Build history of the part. All positions in model axes, mm. A direction names the side the tool comes from. Coordinates: 2 decimals unless noted, no trailing zeros. Write each loop counter-clockwise with the first axis right and the second up, starting at its lowest first coordinate (ties: lowest second). Pieces come first, ordered by that corner, then holes.
```python
from build123d import *

# Parameters (mm, degrees)
BOSS_EXTRUDE1_DEPTH                                 = 15
FILLET1_R                                           = 6
CBORE_FOR_M6_HEX_SOCKET_HEAD_CAP_SCREW1_D           = 6.6
CBORE_FOR_M6_HEX_SOCKET_HEAD_CAP_SCREW1_CBORE_D     = 11
CBORE_FOR_M6_HEX_SOCKET_HEAD_CAP_SCREW1_CBORE_DEPTH = 6.4
SKETCH6_R                                           = 7
CUT_EXTRUDE3_DEPTH                                  = 16
SKETCH7_R                                           = 11
CUT_EXTRUDE4_DEPTH                                  = 11
TAP_DRILL_FOR_M5_TAP1_D                             = 4.2
TAP_DRILL_FOR_M5_TAP1_DEPTH                         = 10
TAP_DRILL_FOR_M5_TAP1_TIP                           = 1.2618073
FILLET4_R                                           = 14
FILLET5_R                                           = 10
CHAMFER1_SIZE                                       = 0.5


with BuildPart() as part:
    # Sketch1 → Boss-Extrude1 (new body)
    with BuildSketch(Plane.XY):
        with BuildLine():
            Line((-54.083500753, -8.556617627), (-54.083500753, -51.556617627))
            Line((-54.083500753, -51.556617627), (-21.808305332, -51.556617627))
            Line((-21.808305332, -51.556617627), (-10.687429148, -20.70518937))
            ThreePointArc((-10.687429148, -20.70518937), (19.416499247, 0.443382373), (49.520427642, -20.70518937))
            Line((49.520427642, -20.70518937), (60.641303826, -51.556617627))
            Line((60.641303826, -51.556617627), (92.916499247, -51.556617627))
            Line((92.916499247, -51.556617627), (92.916499247, 42.193382373))
            Line((92.916499247, 42.193382373), (-74.083500753, 42.193382373))
            Line((-74.083500753, 42.193382373), (-74.083500753, 144.193382373))
            Line((-74.083500753, 144.193382373), (-104.083500753, 144.193382373))
            Line((-104.083500753, 144.193382373), (-104.083500753, 41.443382373))
            Line((-104.083500753, 41.443382373), (-54.083500753, -8.556617627))
        make_face()
        with BuildLine():
            ThreePointArc((-93.483500753, 97.193382373), (-89.083500753, 101.593382373), (-84.683500753, 97.193382373))
            Line((-84.683500753, 97.193382373), (-84.683500753, 85.193382373))
            ThreePointArc((-84.683500753, 85.193382373), (-89.083500753, 80.793382373), (-93.483500753, 85.193382373))
            Line((-93.483500753, 85.193382373), (-93.483500753, 97.193382373))
        make_face(mode=Mode.SUBTRACT)
        with BuildLine():
            ThreePointArc((-93.483500753, 129.193382373), (-89.083500753, 133.593382373), (-84.683500753, 129.193382373))
            Line((-84.683500753, 129.193382373), (-84.683500753, 117.193382373))
            ThreePointArc((-84.683500753, 117.193382373), (-89.083500753, 112.793382373), (-93.483500753, 117.193382373))
            Line((-93.483500753, 117.193382373), (-93.483500753, 129.193382373))
        make_face(mode=Mode.SUBTRACT)
    extrude(amount=BOSS_EXTRUDE1_DEPTH)

    # Fillet1
    fillet1_edges = [part.edges().sort_by_distance(p)[0] for p in [
        (-21.808305332, -51.556617627, 7.5),
        (-54.083500753, -51.556617627, 7.5),
        (-104.083500753, 144.193382373, 7.5),
        (-74.083500753, 144.193382373, 7.5),
        (-74.083500753, 42.193382373, 7.5),
        (60.641303826, -51.556617627, 7.5),
    ]]
    fillet(fillet1_edges, radius=FILLET1_R)

    # CBORE for M6 Hex Socket Head Cap Screw1 (through all)
    with Locations(Plane.XY.offset(15)):
        with Locations((-31.583500753, -41.556617627), (-31.583500753, -21.556617627), (70.416499247, -41.556617627), (70.416499247, -21.556617627)):
            CounterBoreHole(CBORE_FOR_M6_HEX_SOCKET_HEAD_CAP_SCREW1_D / 2, CBORE_FOR_M6_HEX_SOCKET_HEAD_CAP_SCREW1_CBORE_D / 2, CBORE_FOR_M6_HEX_SOCKET_HEAD_CAP_SCREW1_CBORE_DEPTH)

    # Sketch6 → Cut-Extrude3 (cut, through all)
    with BuildSketch(Plane.XY.offset(15)):
        with Locations((78.916499247, 28.193382373)):
            Circle(SKETCH6_R)
    extrude(amount=-CUT_EXTRUDE3_DEPTH, mode=Mode.SUBTRACT)

    # Sketch7 → Cut-Extrude4 (cut)
    with BuildSketch(Plane.XY.offset(15)):
        with Locations((78.916499247, 28.193382373)):
            Circle(SKETCH7_R)
    extrude(amount=-CUT_EXTRUDE4_DEPTH, mode=Mode.SUBTRACT)

    # Tap Drill for M5 Tap1
    with Locations(Plane(origin=(0, 42.193382373, 0), x_dir=(1, 0, 0), z_dir=(0, 1, 0))):
        with Locations((-62.583500753, -7.5)):
            Hole(TAP_DRILL_FOR_M5_TAP1_D / 2, depth=TAP_DRILL_FOR_M5_TAP1_DEPTH)
            with Locations((0, 0, -(TAP_DRILL_FOR_M5_TAP1_DEPTH + TAP_DRILL_FOR_M5_TAP1_TIP / 2))):  # 118° drill point
                Cone(0, TAP_DRILL_FOR_M5_TAP1_D / 2, TAP_DRILL_FOR_M5_TAP1_TIP, mode=Mode.SUBTRACT)

    # Fillet4
    fillet4_edges = [part.edges().sort_by_distance(p)[0] for p in [
        (92.916499247, 42.193382373, 7.5),
    ]]
    fillet(fillet4_edges, radius=FILLET4_R)

    # Fillet5
    fillet5_edges = [part.edges().sort_by_distance(p)[0] for p in [
        (-54.083500753, -8.556617627, 7.5),
        (-104.083500753, 41.443382373, 7.5),
    ]]
    fillet(fillet5_edges, radius=FILLET5_R)

    # Chamfer1
    chamfer1_edges = [part.edges().sort_by_distance(p)[0] for p in [
        (64.916499247, -41.556617627, 15),
        (-37.083500753, -21.556617627, 15),
        (-37.083500753, -41.556617627, 15),
        (67.916499247, 28.193382373, 15),
        (-60.483500753, 42.193382373, 7.5),
        (88.815994184, 38.09287731, 15),
        (-79.083500753, 16.443382373, 15),
        (-104.083500753, 91.889450185, 15),
        (-103.322296078, 41.758683673, 15),
        (-54.844705428, -8.871918927, 15),
        (19.416499247, 0.443382373, 15),
        (54.366178458, -34.148224897, 15),
        (92.916499247, -11.681617627, 15),
        (-74.083500753, 93.193382373, 15),
        (5.416499247, 42.193382373, 15),
        (-89.083500753, 144.193382373, 15),
        (78.886457547, -51.556617627, 15),
        (-54.083500753, -29.127685439, 15),
        (-37.053459053, -51.556617627, 15),
        (-22.574349131, -50.466192801, 15),
        (61.407347625, -50.466192801, 15),
        (-52.32614144, -49.799258314, 15),
        (-102.32614144, 142.43602306, 15),
        (-75.840860066, 142.43602306, 15),
        (-72.32614144, 43.950741686, 15),
        (-15.533179964, -34.148224897, 15),
        (64.916499247, -21.556617627, 15),
    ]]
    chamfer(chamfer1_edges, length=CHAMFER1_SIZE)


solid = part.part
```
1. Flat gauge pins, fed straight in: pin 1 (3 mm diameter, centred on y = 19.5, z = 6, fed in from -X); pin 2 (11 mm diameter, centred on x = 75.5, y = 25.5, fed in from +Z); pin 3 (3.5 mm diameter, centred on x = 72, y = -21, fed in from +Z). Where does each tip first touch, or does it go through?
Computed values:
pin 1: stops at x = -83.64
pin 2: stops at z = 4
pin 3: stops at z = 8.6
2. Probe line 1 along Y through (x, z) = (-30.5, 1.5); line 2 along X through (y, z) = (120, 1.5); line 3 along Y through (x, z) = (73, 8.25). List the from-to ranges inside material, lowest first.
Computed values:
line 1: y = -51.56 to -44.67, -38.44 to -24.67, -18.44 to 42.19
line 2: x = -104.08 to -93.48, -84.68 to -74.08
line 3: y = -51.56 to -43.61, -39.5 to -23.61, -19.5 to 18.92, 37.47 to 42.19
3. Saw through at A-A on x = -45. List the corners of the cut face in (y, z).
Computed values:
outline: (-51.56, 0) - (42.19, 0) - (42.19, 14.5) - (41.69, 15) - (-51.06, 15) - (-51.56, 14.5) - close
4. Mould opens along X. For faces 1 (the face through (-78.6, 16.31, 14.75)), 2 (the face through (-37, -51.557, 7)), 3 (the face through (-89.18, 101.592, 7.395)), 4 (the face through (88.71, 38.2, 7.35)) say: +X half, -X half, draft (parallel to the pull), parting line (faces both ways), or undercut.
Computed values:
face 1: -X half
face 2: draft
face 3: undercut
face 4: +X half
5. 3-axis set-ups, long thin cutter, end or side, ignore diameter. For faces 5 (the face through (-22.62, -50.5, 7.35)), 6 (the face through (-74.084, 93, 7)), 7 (the face through (-64.587, 36.877, 6.869)): which of +Z, -Z, +X, -X, +Y, -Y reach the whole face in a straight line?
Computed values:
face 5: +Z, -Z, -Y
face 6: +Z, -Z, +X, +Y
face 7: +Y
